from build123d import *

# Parameters (mm, degrees)
F0_W     = 25.4
F0_H     = 25.4
F1_DEPTH = 25.4
F2_W     = 25.4
F2_H     = 25.4
F3_DEPTH = 25.4
F4_W     = 25.4
F4_H     = 25.4
F5_DEPTH = 25.4
F6_R     = 25.39999


# Not quite as in the source:
# - a fillet or chamfer is up to 0.001 mm smaller than in the source, because OpenCascade refuses the exact size


with BuildPart() as f1:
    # F0 (on Top) → F1 (new body)
    with BuildSketch(Plane.XY):
        with Locations((12.7, 12.7)):
            Rectangle(F0_W, F0_H)
    extrude(amount=F1_DEPTH)

    # F2 (on face) → F3 (join)
    with BuildSketch(Plane.XY.offset(25.4)):
        Polygon((-25.4, 0), (0, 0), (0, 25.4), (0, 76.2), (-25.4, 76.2), align=None)
        with Locations((12.7, 12.7)):
            Rectangle(F2_W, F2_H)
    extrude(amount=F3_DEPTH)

    # F4 (on face) → F5 (join)
    with BuildSketch(Plane.XY.offset(50.8)):
        with Locations((-12.7, 63.5)):
            Rectangle(F4_W, F4_H)
    extrude(amount=F5_DEPTH)

    # F6 (radius 25.4 in the source; OpenCascade refuses exactly that, so slightly less here)
    f6_edges = [f1.edges().sort_by_distance(p)[0] for p in [
        (12.7, 0, 0),
        (-25.4, 0, 38.1),
        (-25.4, 63.5, 76.2),
        (-12.7, 76.2, 76.2),
        (-25.4, 76.2, 50.8),
    ]]
    fillet(f6_edges, radius=F6_R)


solid = f1.part
Input: part model. Units: mm. Frame: model coordinates. A direction names the side the tool comes from. Give positions to 0.01 mm unless a question says otherwise; leave off trailing zeros. Order: outer loops, then holes, each group sorted by start corner. A loop starts at its lowest first (then second) coordinate and runs counter-clockwise, first axis right, second up. Notation, with made-up numbers: (-7.75, 31) -> (1.25, 31) arc R25 ccw to (1.25, 67) -> close; hole circle Ø10 at (32, -18). An arc over 180 degrees is marked (long way). Use one line per item in the form item = value.
1) Reachability of faces 1 (the flat face through (-6, 26, 50.8)), 2 (the flat face through (0, 15, 15)), 3 (the flat face through (0, 56, 45)) from +Z, -Z, +X, -X, +Y, -Y: full face, straight path, thin tool, end or side. Return the list, or none.
Response values:
face_1 = +Z, +X, -X, -Y
face_2 = -Z, -X, +Y, -Y
face_3 = +Z, -Z, +X, +Y
2) First-contact query: pin 1 Ø20.5 at (x, y) = (-17, 46.5) entering from -Z; pin 2 Ø12 at (x, y) = (-13.5, 15.5) entering from +Z; pin 3 Ø8 at (y, z) = (54.5, 52) entering from +X. Flat tips, straight axial feed; report the tip coordinate or a pass-through.
Response values:
pin_1 = 25.4
pin_2 = 50.8
pin_3 = 0
3) Section C-C, the plane y = 42.5. Return loops of the section in (x, z), and give its area (3 significant figures).
Response values:
outline = (-25.4, 25.4) -> (0, 25.4) -> (0, 50.8) -> (-25.4, 50.8) -> close
area = 645 mm^2
4) Line query: probe 1 along Z at (x, y) = (-19.5, 41.5); probe 2 along Y at (x, z) = (21, 43.5). Output: solid intervals per line, ascending.
Response values:
probe_1 = 25.4 to 50.8
probe_2 = 0 to 25.4
